The model under review builds one solid part; all positions refer to its coordinate system, in mm. A direction names the side the tool comes from. Give positions to 0.01 mm unless a question says otherwise; leave off trailing zeros. Write each loop counter-clockwise with the first axis right and the second up, starting at its lowest first coordinate (ties: lowest second). Pieces come first, ordered by that corner, then holes. Notation, with made-up numbers: (-25.75, 89) -> (-8.75, 89) arc R11 ccw to (-8.75, 93) -> close; hole circle Ø6 at (89.25, 78.25). An arc over 180 degrees is marked (long way). Use CSV: the item, a comma, the result in double quotes.
```python
from build123d import *

# Parameters (mm, degrees)
F0_W     = 55
F0_H     = 32
F1_DEPTH = 40
F2_W     = 30
F2_H     = 18
F3_DEPTH = 20
F4_R     = 5
F5_DEPTH = 20.001
F6_SIZE  = 2
F7_R     = 3


with BuildPart() as f1:
    # F0 (on Front) → F1 (new body)
    with BuildSketch(Plane.XZ):
        with Locations((27.5, -16)):
            Rectangle(F0_W, F0_H)
    extrude(amount=F1_DEPTH)

    # F2 (on face) → F3 (cut)
    with BuildSketch(Plane.XZ.offset(40)):
        with Locations((40, -23)):
            Rectangle(F2_W, F2_H)
    extrude(amount=-F3_DEPTH, mode=Mode.SUBTRACT)

    # F4 (on face) → F5 (cut, through all)
    with BuildSketch(Plane.XZ.offset(20)):
        with Locations((41.2149988763, -23.5055347287)):
            Circle(F4_R)
    extrude(amount=-F5_DEPTH, mode=Mode.SUBTRACT)

    # F6
    f6_edges = [f1.edges().sort_by_distance(p)[0] for p in [
        (0, -20, -32),
        (25, -30, -32),
        (25, -30, -14),
        (55, -20, 0),
        (55, -30, -14),
        (0, -20, 0),
    ]]
    chamfer(f6_edges, length=F6_SIZE)

    # F7
    f7_edges = [f1.edges().sort_by_distance(p)[0] for p in [
        (25, -40, -23),
        (24, -40, -31),
        (12.5, -40, -32),
        (0, -40, -16),
        (55, -40, -7),
        (54, -40, -13),
        (54, -40, -1),
        (40, -40, -14),
        (27.5, -40, 0),
        (26, -40, -15),
        (1, -40, -1),
        (1, -40, -31),
    ]]
    fillet(f7_edges, radius=F7_R)


solid = f1.part
```
Q1. Consider section A-A (x = 50.5). Write out the cut boundary in (y, z).
Derived:
outline,"(-40, -11) arc R3 ccw to (-37, -14) -> (-20, -14) -> (-20, -32) -> (0, -32) -> (0, 0) -> (-37, 0) arc R3 ccw to (-40, -3) -> close"
Q2. Consider section C-C (z = -25.5). Write out the cut boundary in (x, y).
Derived:
outline,"(0, -37) arc R3 ccw to (3, -40) -> (22, -40) arc R3 ccw to (25, -37) -> (25, -20) -> (36.63, -20) -> (36.63, 0) -> (0, 0) -> close; (45.8, -20) -> (55, -20) -> (55, 0) -> (45.8, 0) -> close"
Q3. Consider section D-D (y = -9). Write out the cut boundary in (x, z) (3 decimals).
Derived:
outline,"(0, -30) -> (2, -32) -> (55, -32) -> (55, -2) -> (53, 0) -> (2, 0) -> (0, -2) -> close; hole circle Ø10 at (41.215, -23.506)"
Q4. Consider section B-B (y = -28.5). Write out the cut boundary in (x, z), then the cut area to 3 significant figures.
Derived:
outline,"(0, -30) -> (2, -32) -> (23, -32) -> (25, -30) -> (25, -16) -> (27, -14) -> (53, -14) -> (55, -12) -> (55, -2) -> (53, 0) -> (2, 0) -> (0, -2) -> close"
area,"1,210 mm2"
Q5. Insertion check: pin 1 (5 mm diameter, centred on y = -26.5, z = -19.5, fed in from +X); pin 2 (5 mm diameter, centred on x = 42.5, y = -24.5, fed in from -Z); pin 3 (16 mm diameter, centred on x = 47, z = -22.5, fed in from -Y). Each pin has a flat end and moves straight along its axis. Give the tip position at first contact, or say it passes through.
Derived:
pin 1,"stops at x = 25"
pin 2,"stops at z = -14"
pin 3,"stops at y = -20"
Q6. To check wall thickness, follow probe 1 along Z at (x, y) = (29.5, -20.5); probe 2 along X at (y, z) = (-11, -23); probe 3 along Y at (x, z) = (38, -30.5). State the ranges of each line that lie inside material, in increasing order.
Derived:
probe 1,"z = -14 to 0"
probe 2,"x = 0 to 36.24, 46.19 to 55"
probe 3,"y = -20 to 0"
Q7. The part is to be moulded in two halves that separate along Z. For faces 3 (the cylindrical face through (37.25, -10.14, -26.55)), 4 (the flat face through (35, -20, -24)), 5 (the cylindrical face through (1.411, -38.748, -1.383)), 6 (the cylindrical face through (53.589, -38.748, -12.617)), say which applies: pulls with the +Z half, pulls with the -Z half, needs draft (parallel to the pull), parting line crosses it, or undercut.
Derived:
face 3,"undercut"
face 4,"needs draft"
face 5,"pulls with the +Z half"
face 6,"pulls with the -Z half"
Q8. Machinability: for faces 1 (the flat face through (1, -18, -1)), 2 (the flat face through (24, -29, -31)), which of the approach directions +Z, -Z, +X, -X, +Y, -Y give a long, thin tool a straight path to every point of the face, cutting with its end or side? Answer none if there is none.
Derived:
face 1,"+Z, -X, +Y, -Y"
face 2,"-Z, +X, -Y"
